Work out the finished part from the listing and answer in its coordinate system (mm). A direction names the side the tool comes from. Give positions to 0.01 mm unless a question says otherwise; leave off trailing zeros. Order: outer loops, then holes, each group sorted by start corner. A loop starts at its lowest first (then second) coordinate and runs counter-clockwise, first axis right, second up.
Autodesk Fusion 360 part; units mm, degrees
sketch "Sketch1" plane through (0, 0, 0) normal (0, 1, 0) x (1, 0, 0)
  line L0 (0, 0) -> (30, 0)
  line L1 (30, 0) -> (30, -8.5)
  line L2 (30, -8.5) -> (0, -8.5)
  line L3 (0, -8.5) -> (0, 0)
  dimension "d1" = 30
  dimension "d2" = 8.5
extrude "Extrude1" add sketch "Sketch1" along normal blind 6.25
sketch "Sketch2" plane through (0, 0, 0) normal (-1, 0, 0) x (0, -1, 0)
  line L0 (0, 0) -> (0, 8.5)
  line L1 (0, 8.5) -> (-6.25, 8.5)
  line L2 (-6.25, 8.5) -> (-6.25, 0)
  line L3 (-6.25, 0) -> (0, 0)
  line L4 (-6.25, 8.5) -> (-4.375, 8.5)
  line L5 (-4.375, 8.5) -> (-4.375, 6.5)
  line L6 (-4.375, 6.5) -> (-1.875, 6.5)
  line L7 (-1.875, 6.5) -> (-1.875, 2)
  line L8 (-1.875, 2) -> (-4.375, 2)
  line L9 (-4.375, 2) -> (-4.375, 6.5)
  dimension "d5" = 1.875
  dimension "d6" = 2
  dimension "d7" = 2.5
  dimension "d8" = 4.5
extrude "Extrude2" cut sketch "Sketch2" against normal blind 24 contours L6 L7 L8 L9
sketch "Sketch3" plane through (30, 0, 0) normal (1, 0, 0) x (0, 1, 0)
  line L0 (0, 8.5) -> (0, 0)
  line L1 (0, 0) -> (6.25, 0)
  line L2 (6.25, 0) -> (6.25, 8.5)
  line L3 (6.25, 8.5) -> (0, 8.5)
  line L4 (0, 8.5) -> (2.25, 8.5)
  line L5 (2.25, 8.5) -> (2.25, 6.25)
  line L6 (2.25, 6.25) -> (6.25, 6.25)
  line L7 (6.25, 6.25) -> (6.25, 2.25)
  line L8 (6.25, 2.25) -> (2.25, 2.25)
  line L9 (2.25, 2.25) -> (2.25, 6.25)
  dimension "d11" = 2.25
  dimension "d12" = 2.25
  dimension "d13" = 4
  dimension "d14" = 4
extrude "Extrude3" add sketch "Sketch3" along normal blind 30 contours L2 L6 L7 L8 L9
1. The mould has two halves that part along Y. Classify faces 1 (the face through (30, 2, 4)), 2 (the face through (15, 0, 4)), 3 (the face through (12, 3, 2)): pulls with the +Y half, pulls with the -Y half, needs draft (parallel to the pull), parting line crosses it, or undercut.
Findings below:
face 1: needs draft
face 2: pulls with the -Y half
face 3: undercut
2. The part is cut by section B-B (z = 3.75). Write down the section's boundary in (x, y) (3 decimals), then the cut area to 4 significant figures.
Findings below:
outline: (0, 0) - (30, 0) - (30, 2.25) - (60, 2.25) - (60, 6.25) - (0, 6.25) - (0, 4.375) - (24, 4.375) - (24, 1.875) - (0, 1.875) - close
area: 247.5 mm2
3. The part is cut by section D-D (x = 45). Write down the section's boundary in (y, z).
Findings below:
outline: (2.25, 2.25) - (6.25, 2.25) - (6.25, 6.25) - (2.25, 6.25) - close
4. Which of the six approach directions +Z, -Z, +X, -X, +Y, -Y give full straight-line access (tool end or side, diameter ignored) to faces 4 (the face through (45, 4, 6.25)), 5 (the face through (15, 3, 8.5)), 6 (the face through (45, 4, 2.25)), 7 (the face through (24, 3, 4)), 8 (the face through (45, 2.25, 4))?
Findings below:
face 4: +Z, +X, +Y, -Y
face 5: +Z, +X, -X, +Y, -Y
face 6: -Z, +X, +Y, -Y
face 7: -X
face 8: +Z, -Z, +X, -Y
5. The part is cut by section C-C (y = 3.5). Write down the section's boundary in (x, z), then the cut area to 3 significant figures.
Findings below:
outline: (0, 0) - (30, 0) - (30, 2.25) - (60, 2.25) - (60, 6.25) - (30, 6.25) - (30, 8.5) - (0, 8.5) - (0, 6.5) - (24, 6.5) - (24, 2) - (0, 2) - close
area: 267 mm2
6. Given P1, Ø0.8, axis at y = 2.5, z = 5, coming from the -X side; P2, Ø1.2, axis at x = 42, y = 4.5, coming from the -Z side; P3, Ø2, axis at x = 48.5, z = 4, coming from the -Y side, each flat-ended and moving along its own axis, determine where each tip first touches the part or whether it passes through.
Findings below:
P1: stops at x = 24
P2: stops at z = 2.25
P3: stops at y = 2.25
7. The part is cut by section A-A (x = 17). Write down the section's boundary in (y, z) (3 decimals).
Findings below:
outline: (0, 0) - (6.25, 0) - (6.25, 8.5) - (0, 8.5) - close; hole (1.875, 2) - (4.375, 2) - (4.375, 6.5) - (1.875, 6.5) - close
8. Straight lines are drawn through the part: probe 1 along Z at (x, y) = (5.5, 3.25); probe 2 along X at (y, z) = (2.25, 1.5); probe 3 along Y at (x, z) = (7.5, 4.25) (3 decimals). For each, find the intervals that lie inside material, in ascending order.
Findings below:
probe 1: z = 0 to 2, 6.5 to 8.5
probe 2: x = 0 to 30
probe 3: y = 0 to 1.875, 4.375 to 6.25
